The listing builds one solid part. Answer for the finished solid, in the listing's coordinates (mm). Face numbers are marked on the shaded views. A direction names the side the tool comes from. Round coordinates to 2 decimals unless told otherwise and drop trailing zeros. Order: outer loops, then holes, each group sorted by start corner. A loop starts at its lowest first (then second) coordinate and runs counter-clockwise, first axis right, second up. Notation, with made-up numbers: M 3.5,38 L 60.5,38 A9 ccw 60.5,49 Z; hole C 54.25,33 d5. An arc over 180 degrees is marked long. Write item = value, one per line. Start each with the question number.
(1) A cutting plane is placed at C-C, the plane z = 0. Determine the outline of the cut face in (x, y), and give its area (3 significant figures).
(2) For a pull along X with two mould halves and no side action, classify the marked faces 3, 4, 5 and 6 as released by +X, released by -X, zero draft, split by the parting line, or undercut.
(3) Straight lines are drawn through the part: probe 1 along Z at (x, y) = (0, -13.25); probe 2 along Z at (x, y) = (12, -26.5); probe 3 along Y at (x, z) = (94, -7). For each, find the intervals that lie inside material, in ascending order. Write a range as from..to.
(4) A cutting plane is placed at D-D, the plane z = 23. Determine the outline of the cut face in (x, y), and give its area (3 significant figures).
(5) A cutting plane is placed at A-A, the plane x = 88. Determine the outline of the cut face in (y, z).
(6) Which of the six approach directions +Z, -Z, +X, -X, +Y, -Y give full straight-line access (tool end or side, diameter ignored) to the marked faces 1 and 2?
(7) Each of these flat-tipped pins is pushed along its axis until it touches: pin 1 (4 mm diameter, centred on y = -13, z = -3.5, fed in from -X); pin 2 (8 mm diameter, centred on y = -30.5, z = -58, fed in from -X); pin 3 (3 mm diameter, centred on y = -31.5, z = -21.5, fed in from -X); pin 4 (3 mm diameter, centred on x = 159.5, z = 7, fed in from +Y). Where does it stop, or does it pass through?
(8) A cutting plane is placed at B-B, the plane y = -26.5. Determine the outline of the cut face in (x, z).
from build123d import *

# Parameters (mm, degrees)
F1_DEPTH = 35
F4_DEPTH = 19
F5_R     = 26
F6_DEPTH = 15


with BuildPart() as f1:
    # F0 (on Front) → F1 (new body)
    with BuildSketch(Plane.XZ):
        with BuildLine():
            Line((111, 76), (0, 76))
            ThreePointArc((0, 76), (-76, 0), (0, -76))
            Line((0, -76), (111, -76))
            ThreePointArc((111, -76), (187, 0), (111, 76))
        make_face()
    extrude(amount=F1_DEPTH)

    # F3 (on offset) → F4 (cut)
    with BuildSketch(Plane.XZ.offset(19)):
        with BuildLine():
            Line((111, 64), (0, 64))
            ThreePointArc((0, 64), (-64, 0), (0, -64))
            Line((0, -64), (111, -64))
            ThreePointArc((111, -64), (175, 0), (111, 64))
        make_face()
    extrude(amount=F4_DEPTH, mode=Mode.SUBTRACT)

    # F5 (on offset) → F6 (cut)
    with BuildSketch(Plane.XZ.offset(19)):
        Circle(F5_R)
    extrude(amount=-F6_DEPTH, mode=Mode.SUBTRACT)


solid = f1.part
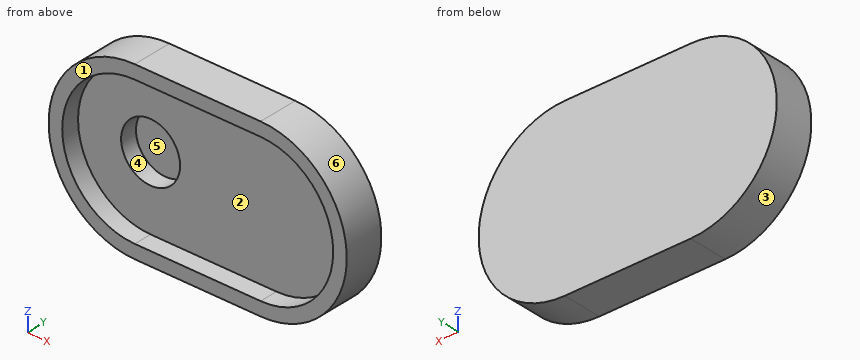
Reported:
q1.outline = M -76,-35 L -64,-35 L -64,-19 L -26,-19 L -26,-4 L 26,-4 L 26,-19 L 175,-19 L 175,-35 L 187,-35 L 187,0 L -76,0 Z
q1.area = 4,600 mm²
q2.face_3 = released by -X
q2.face_4 = undercut
q2.face_5 = undercut
q2.face_6 = released by +X
q3.probe_1 = -76..-26, 26..76
q3.probe_2 = -76..-64, 64..76
q3.probe_3 = -19..0
q4.outline = M -72.44,-35 L -59.72,-35 L -59.72,-19 L -12.12,-19 L -12.12,-4 L 12.12,-4 L 12.12,-19 L 170.72,-19 L 170.72,-35 L 183.44,-35 L 183.44,0 L -72.44,0 Z
q4.area = 4,900 mm²
q5.outline = M -35,-76 L 0,-76 L 0,76 L -35,76 L -35,64 L -19,64 L -19,-64 L -35,-64 Z
q6.face_1 = +Z, -Z, +X, -X, -Y
q6.face_2 = -Y
q7.pin_1 = -75.99
q7.pin_2 = -53.48
q7.pin_3 = -73.32
q7.pin_4 = 0
q8.outline = M 0,-76 L 111,-76 A76 ccw 111,76 L 0,76 A76 ccw Z; hole M 0,-64 L 111,-64 A64 ccw 111,64 L 0,64 A64 ccw Z
